Can you work these out from the model? Positions are in its coordinate system, mm. A direction names the side the tool comes from. Give positions to 0.01 mm unless a question says otherwise; leave off trailing zeros. Order: outer loops, then holes, each group sorted by start corner. A loop starts at its lowest first (then second) coordinate and runs counter-clockwise, first axis right, second up. Notation, with made-up numbers: (-28.5, -17) -> (-23.5, -17) arc R14 cw to (-23.5, -11) -> close; hole circle Ø3 at (80.5, 66.25). An arc over 180 degrees is marked (long way). Answer as a JSON object with one key per item and string values.
Autodesk Inventor part; units mm, degrees
ref_plane "Work Plane1" through (-33.6677, 0, 3.175) normal (0, 1, 0) x (1, 0, 0)
ref_plane "YZ Plane" through (0, 0, 0) normal (1, 0, 0) x (0, 1, 0)
ref_plane "XZ Plane" through (0, 0, 0) normal (0, 1, 0) x (-1, 0, 0)
sketch "Sketch1" plane through (0, 0, 0) normal (0, 0, 1) x (1, 0, 0)
  circle A0 centre (0, 0) radius 14.2875
  line L0 (-33.6677, 0) -> (-23.1902, 0) construction
  line L1 (-33.6677, -2.5527) -> (-23.1902, -2.5527)
  line L2 (-23.1902, 2.5527) -> (-33.6677, 2.5527)
  arc A1 (-33.6677, 2.5527) -> (-33.6677, -2.5527) centre (-33.6677, 0) ccw
  arc A2 (-23.1902, -2.5527) -> (-23.1902, 2.5527) centre (-23.1902, 0) ccw
  line L3 (23.1902, 0) -> (33.6677, 0) construction
  line L4 (23.1902, -2.5527) -> (33.6677, -2.5527)
  line L5 (33.6677, 2.5527) -> (23.1902, 2.5527)
  arc A3 (23.1902, 2.5527) -> (23.1902, -2.5527) centre (23.1902, 0) ccw
  arc A4 (33.6677, -2.5527) -> (33.6677, 2.5527) centre (33.6677, 0) ccw
  line L6 (-14.2875, 17.4625) -> (-39.3954, 6.35)
  line L7 (-39.3954, 6.35) -> (-39.3954, -6.35)
  line L8 (-39.3954, -6.35) -> (-14.2875, -17.4625)
  line L9 (-14.2875, -17.4625) -> (14.2875, -17.4625)
  line L10 (14.2875, -17.4625) -> (39.3954, -6.35)
  line L11 (39.3954, -6.35) -> (39.3954, 6.35)
  line L12 (39.3954, 6.35) -> (14.2875, 17.4625)
  line L13 (14.2875, 17.4625) -> (-14.2875, 17.4625)
  circle A5 centre (-23.1902, 0) radius 4.7625 construction
  circle A6 centre (0, 0) radius 13.6398 construction
  circle A7 centre (-45.9552, 70.4429) radius 54.5719 construction
  circle A8 centre (-1.8189, -39.1868) radius 18.1864 construction
  line L14 (8.4839, 74.2476) -> (16.3232, -37.9189) construction
  line L15 (-15.7788, -50.843) -> (-87.8447, 35.4663) construction
  line L16 (-45.9552, 70.4429) -> (4.7485, 67.3163) construction
  line L17 (4.7485, 67.3163) -> (-1.8189, -39.1868) construction
  point P0 (-28.429, 0)
  point P1 (28.429, 0)
  point P2 (0, 17.4625)
  point P3 (0, 14.2875)
  point P4 (-20.6375, 0)
  point P5 (-14.2875, 0)
  point P6 (-36.2204, 0)
  point P7 (-39.3954, 0)
  point P8 (39.3954, 0)
  dimension "d0" = 28.575
  dimension "d3" = 28.575
  dimension "d4" = 3.175
  dimension "d5" = 17.4625
  dimension "d6" = 17.4625
  dimension "d7" = 10.4775
  dimension "d8" = 10.4775
  dimension "d9" = 6.35
  dimension "d10" = 5.1054
  dimension "d11" = 28.429
  dimension "d12" = 9.525
  dimension "d13" = 27.2796
  dimension "d16" = 109.1438
  dimension "d19" = 36.3728
  dimension "d20" = 106.7054
  dimension "d21" = 50.8
  dimension "d22" = 28.429
  dimension "d23" = 3.175
  dimension "d24" = 5.7277
  dimension "d25" = 5.7277
  dimension "d26" = 12.7
extrude "Extrusion1" add sketch "Sketch1" along normal mid plane 6.35
fillet "Fillet1" radius 6.35 8 edges at (-14.2875, 17.4625, 0) (14.2875, 17.4625, 0) (39.3954, 6.35, 0) (39.3954, -6.35, 0) (14.2875, -17.4625, 0) (-14.2875, -17.4625, 0) (-39.3954, -6.35, 0) (-39.3954, 6.35, 0)
ref_plane "Work Plane1" through (-33.6677, 0, 3.175) normal (0, 1, 0) x (1, 0, 0)
equation "\"d6\" = d5"
properties part number "EL2-CGB-010" material "Aluminum 6061"
1. Will these pins go through, and if not, where does the flat tip stop? pin 1 Ø2 at (y, z) = (4, -2) entering from +X; pin 2 Ø3 at (x, z) = (27, 0.5) entering from +Y; pin 3 Ø1.9 at (x, z) = (29.5, -1.5) entering from -Y.
Worked answers:
{"pin 1": "x = 39.35", "pin 2": "y = 12.5", "pin 3": "y = -11.15"}
2. If we section it at D-D on y = 0: Please give me the cut outline in (x, z) (1 decimal).
Worked answers:
{"outline": "(-39.4, -3.2) -> (-36.2, -3.2) -> (-36.2, 3.2) -> (-39.4, 3.2) -> close; (-20.6, -3.2) -> (-14.3, -3.2) -> (-14.3, 3.2) -> (-20.6, 3.2) -> close; (14.3, -3.2) -> (20.6, -3.2) -> (20.6, 3.2) -> (14.3, 3.2) -> close; (36.2, -3.2) -> (39.4, -3.2) -> (39.4, 3.2) -> (36.2, 3.2) -> close"}
3. For faces 4 (the face through (-9, 12, -3.175)), 5 (the face through (28, -2.553, 0)), which set-ups out of +Z, -Z, +X, -X, +Y, -Y let a thin tool reach every point of the face, with its end or its side?
Worked answers:
{"face 4": "-Z, +X, -X, +Y, -Y", "face 5": "+Z, -Z"}
4. If we section it at C-C on y = -9: Please give me the cut outline in (x, z) (3 decimals).
Worked answers:
{"outline": "(-33.408, -3.175) -> (-11.097, -3.175) -> (-11.097, 3.175) -> (-33.408, 3.175) -> close; (11.097, -3.175) -> (33.408, -3.175) -> (33.408, 3.175) -> (11.097, 3.175) -> close"}
5. Please list where these lines run through material, in increasing order: L1, parallel to Y at x = 0, z = 1.25; L2, parallel to X at y = 8.5, z = -0.5; L3, parallel to X at y = -8, z = -0.25.
Worked answers:
{"L1": "-17.46 to -14.29, 14.29 to 17.46", "L2": "-34.54 to -11.48, 11.48 to 34.54", "L3": "-35.67 to -11.84, 11.84 to 35.67"}
6. If we mould it in two halves opening along Y, with no side actions, what happens to faces 1 (the face through (38.34, 5.72, -0.04)), 2 (the face through (20.64, -0.06, -0.04)), 3 (the face through (14.28, -17.32, -0.04))? For each: +Y half, -Y half, draft (parallel to the pull), parting line (faces both ways), or undercut.
Worked answers:
{"face 1": "+Y half", "face 2": "undercut", "face 3": "-Y half"}
7. If we section it at B-B on z = -1.75: Count the separate pieces of the cut face and the enclosed holes in it, then the cut area to 3 significant figures.
Worked answers:
{"separate pieces": "1", "enclosed holes": "3", "area": "1,390 mm²"}
8. If we section it at A-A on x = 0: Please give me the cut outline in (y, z) (1 decimal).
Worked answers:
{"outline": "(-17.5, -3.2) -> (-14.3, -3.2) -> (-14.3, 3.2) -> (-17.5, 3.2) -> close; (14.3, -3.2) -> (17.5, -3.2) -> (17.5, 3.2) -> (14.3, 3.2) -> close"}
